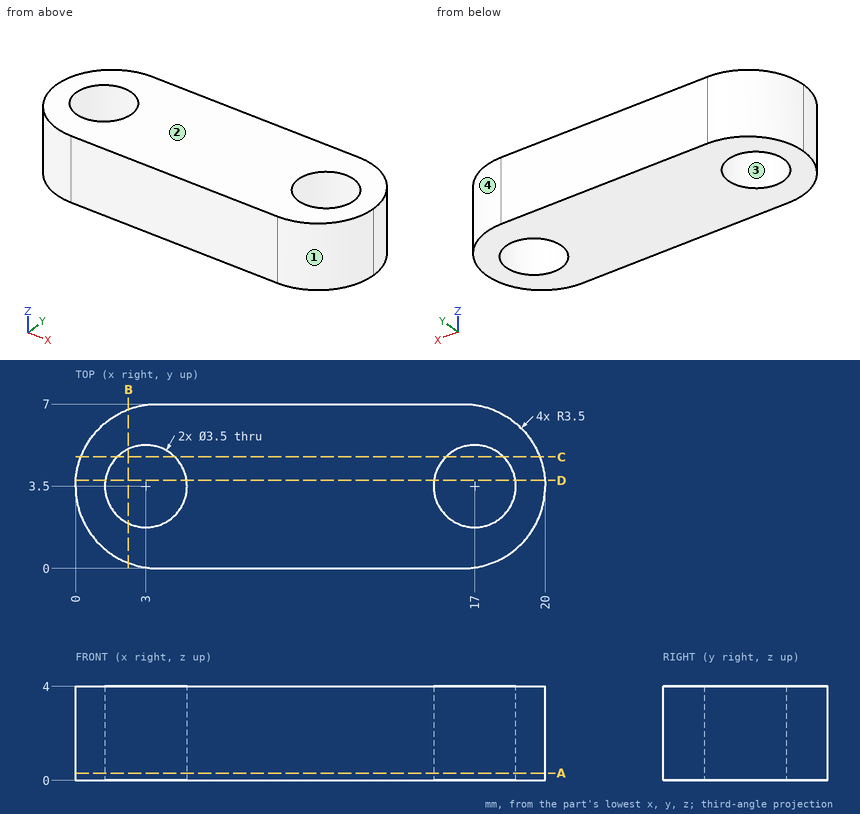
Check sheet for the drawn part. Datum: minimum x, y, z corner. Units: mm. Give positions to 0.01 mm unless a question says otherwise; leave off trailing zeros. Loops run counter-clockwise (first coordinate to the right, second up) from the corner with the lowest first, then second, coordinate; pieces in that order, holes last.
1) Sectioned sample at D-D, the plane y = 3.75. Enter the section's corners in (x, z), then the cut area to 3 significant figures.
2) Draft check along Y on the marked faces 1, 2, 3 and 4. Enter one of: pulls with the +Y half, pulls with the -Y half, needs draft (parallel to the pull), parting line crosses it, or undercut.
3) Thickness scan on line 1 along X through (y, z) = (4.25, 1.5); line 2 along X through (y, z) = (2, 2.15); line 3 along Y through (x, z) = (17, 2.95). Record the ranges inside material, lowest first.
4) Sectioned sample at C-C, the plane y = 4.75. Enter the section's corners in (x, z).
5) Depth check by flat-ended pin: pin 1 Ø1 at (y, z) = (2, 1.5) entering from -X; pin 2 Ø3 at (x, y) = (3, 3.5) entering from -Z; pin 3 Ø1 at (y, z) = (2, 3) entering from +X; pin 4 Ø1.5 at (y, z) = (2.5, 3) entering from -X. Enter the tip coordinate at first touch or a pass-through.
6) Sectioned sample at A-A, the plane z = 0.3. Count the separate pieces of the cut face and the enclosed holes in it, then the cut area to 3 significant figures.
7) Sectioned sample at B-B, the plane x = 2.25. Enter the section's corners in (y, z).
Answers:
1. outline: (0.01, 0) - (1.27, 0) - (1.27, 4) - (0.01, 4) - close; (4.73, 0) - (15.27, 0) - (15.27, 4) - (4.73, 4) - close; (18.73, 0) - (19.99, 0) - (19.99, 4) - (18.73, 4) - close
1. area: 52.2 mm2
2. face 1: pulls with the -Y half
2. face 2: needs draft
2. face 3: undercut
2. face 4: pulls with the +Y half
3. line 1: x = 0.08 to 1.42, 4.58 to 15.42, 18.58 to 19.92
3. line 2: x = 0.34 to 2.1, 3.9 to 16.1, 17.9 to 19.66
3. line 3: y = 0.04 to 1.75, 5.25 to 6.96
4. outline: (0.23, 0) - (1.78, 0) - (1.78, 4) - (0.23, 4) - close; (4.22, 0) - (15.78, 0) - (15.78, 4) - (4.22, 4) - close; (18.22, 0) - (19.77, 0) - (19.77, 4) - (18.22, 4) - close
5. pin 1: stops at x = 0.15
5. pin 2: passes through
5. pin 3: stops at x = 19.85
5. pin 4: stops at x = 0.01
6. separate pieces: 1
6. enclosed holes: 2
6. area: 110 mm2
7. outline: (0.23, 0) - (1.92, 0) - (1.92, 4) - (0.23, 4) - close; (5.08, 0) - (6.77, 0) - (6.77, 4) - (5.08, 4) - close
